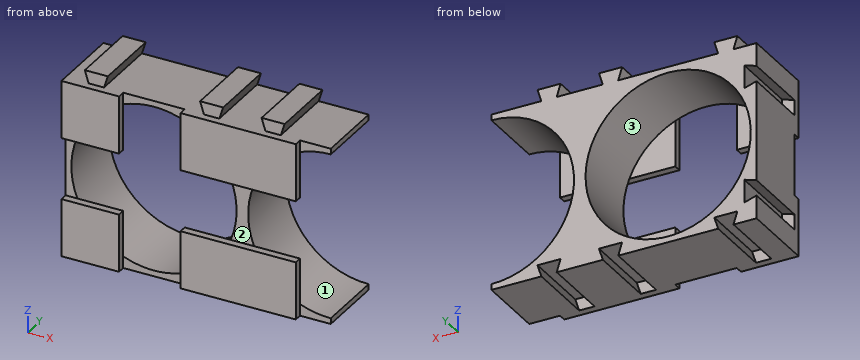
from build123d import *

# Parameters (mm, degrees)
SKETCH1_W           = 47.6
SKETCH1_H           = 24.6
BOSS_EXTRUDE1_DEPTH = 10
SKETCH2_R           = 10.75
CUT_EXTRUDE1_DEPTH  = 9
CUT_EXTRUDE2_DEPTH  = 9
SKETCH5_W           = 1.6
SKETCH5_H           = 24.6
CUT_EXTRUDE3_DEPTH  = 10
SKETCH6_W           = 46
SKETCH6_H           = 1.6
CUT_EXTRUDE4_DEPTH  = 10
BOSS_EXTRUDE2_DEPTH = 9
SKETCH10_W          = 46
SKETCH10_H          = 8.003908937
CUT_EXTRUDE5_DEPTH  = 1
SKETCH11_W          = 8
SKETCH11_H          = 23
CUT_EXTRUDE6_DEPTH  = 1
SKETCH12_W          = 13.355704333
SKETCH12_H          = 24.6
CUT_EXTRUDE8_DEPTH  = 10


with BuildPart() as part:
    # Sketch1 → Boss-Extrude1 (new body)
    with BuildSketch(Plane(origin=(0, 0, 0), x_dir=(1, 0, 0), z_dir=(0, 1, 0))):
        with Locations((23.8, 12.3)):
            Rectangle(SKETCH1_W, SKETCH1_H)
    extrude(amount=BOSS_EXTRUDE1_DEPTH)

    # Sketch2 → Cut-Extrude1 (cut)
    with BuildSketch(Plane(origin=(0, 10, 0), x_dir=(1, 0, 0), z_dir=(0, 1, 0))):
        with Locations(Location((11.5, 13.1, 0), (0, 0, 270))):
            Circle(SKETCH2_R)
        with Locations(Location((34.5, 13.1, 0), (0, 0, 270))):
            Circle(SKETCH2_R)
    extrude(amount=-CUT_EXTRUDE1_DEPTH, mode=Mode.SUBTRACT)

    # Sketch3 → Cut-Extrude2 (cut)
    with BuildSketch(Plane(origin=(0, 10, 0), x_dir=(1, 0, 0), z_dir=(0, 1, 0))):
        Polygon((3, 24.6), (2.5, 23), (5.5, 23), (5, 24.6), align=None)
        Polygon((18, 24.6), (17.5, 23), (20.5, 23), (20, 24.6), align=None)
        Polygon((26, 24.6), (25.5, 23), (28.5, 23), (28, 24.6), align=None)
        Polygon((41, 24.6), (40.5, 23), (43.5, 23), (43, 24.6), align=None)
        Polygon((0, 21.6), (1.6, 22.1), (1.6, 19.1), (0, 19.6), align=None)
        Polygon((0, 6.6), (1.6, 7.1), (1.6, 4.1), (0, 4.6), align=None)
    extrude(amount=-CUT_EXTRUDE2_DEPTH, mode=Mode.SUBTRACT)

    # Sketch5 → Cut-Extrude3 (cut)
    with BuildSketch(Plane(origin=(0, 10, 0), x_dir=(1, 0, 0), z_dir=(0, 1, 0))):
        with Locations((46.8, 12.3)):
            Rectangle(SKETCH5_W, SKETCH5_H)
    extrude(amount=-CUT_EXTRUDE3_DEPTH, mode=Mode.SUBTRACT)

    # Sketch6 → Cut-Extrude4 (cut)
    with BuildSketch(Plane(origin=(0, 10, 0), x_dir=(1, 0, 0), z_dir=(0, 1, 0))):
        with Locations((23, 0.8)):
            Rectangle(SKETCH6_W, SKETCH6_H)
    extrude(amount=-CUT_EXTRUDE4_DEPTH, mode=Mode.SUBTRACT)

    # Sketch7 → Boss-Extrude2 (add)
    with BuildSketch(Plane(origin=(0, 10, 0), x_dir=(1, 0, 0), z_dir=(0, 1, 0))):
        Polygon((46, 21.6), (47.6, 22.1), (47.6, 19.1), (46, 19.6), align=None)
        Polygon((46, 6.6), (47.6, 7.1), (47.6, 4.1), (46, 4.6), align=None)
        Polygon((3, 1.6), (2.5, 0), (5.5, 0), (5, 1.6), align=None)
        Polygon((18, 1.6), (17.5, 0), (20.5, 0), (20, 1.6), align=None)
        Polygon((26, 1.6), (25.5, 0), (28.5, 0), (28, 1.6), align=None)
        Polygon((41, 1.6), (40.5, 0), (43.5, 0), (43, 1.6), align=None)
    extrude(amount=-BOSS_EXTRUDE2_DEPTH)

    # Sketch10 → Cut-Extrude5 (cut)
    with BuildSketch(Plane.XZ):
        with Locations((23, -13.101954469)):
            Rectangle(SKETCH10_W, SKETCH10_H)
    extrude(amount=-CUT_EXTRUDE5_DEPTH, mode=Mode.SUBTRACT)

    # Sketch11 → Cut-Extrude6 (cut)
    with BuildSketch(Plane.XZ):
        with Locations((11.5, -13.1)):
            Rectangle(SKETCH11_W, SKETCH11_H)
        with Locations((34.5, -13.1)):
            Rectangle(SKETCH11_W, SKETCH11_H)
    extrude(amount=-CUT_EXTRUDE6_DEPTH, mode=Mode.SUBTRACT)

    # Sketch12 → Cut-Extrude8 (cut)
    with BuildSketch(Plane(origin=(0, 10, 0), x_dir=(1, 0, 0), z_dir=(0, 1, 0))):
        with Locations((41.177852167, 12.3)):
            Rectangle(SKETCH12_W, SKETCH12_H)
    extrude(amount=-CUT_EXTRUDE8_DEPTH, mode=Mode.SUBTRACT)


solid = part.part
Design review of the part built by this model. Coordinates are the model's own, in mm. Face numbers are marked on the shaded views. A direction names the side the tool comes from. Round coordinates to 2 decimals unless told otherwise and drop trailing zeros. Write each loop counter-clockwise with the first axis right and the second up, starting at its lowest first coordinate (ties: lowest second). Pieces come first, ordered by that corner, then holes.
Item 1: For the marked faces 1, 2 and 3, list the 3-axis set-ups (+Z, -Z, +X, -X, +Y, -Y) from which the entire face can be reached by the end or side of a thin tool; tool diameter is ignored.
Item 2: Consider section C-C on z = -1.25. Give the boundary of the cut face in (x, y), and give its area (3 significant figures).
Item 3: Wall thickness on L1, parallel to X at y = 5, z = -13.1; L2, parallel to X at y = 6, z = -17; L3, parallel to Z at x = 30.5, y = 6: over which ranges is each line inside the solid? List them lowest first.
Item 4: Consider section D-D on x = 6. Give the boundary of the cut face in (y, z), and give its area (3 significant figures).
Item 5: Consider section B-B on z = -13.1. Give the boundary of the cut face in (x, y), and give its area (4 significant figures).
Item 6: Consider section A-A on x = 11.5. Give the boundary of the cut face in (y, z).
Item 7: For pin 1 Ø1.5 at (x, z) = (22.5, -12) entering from -Y; pin 2 Ø0.5 at (x, z) = (0.5, -20.5) entering from +Y; pin 3 Ø0.5 at (y, z) = (0.5, -22) entering from +X; pin 4 Ø2 at (x, z) = (12.5, -4) entering from +Y, all flat-tipped, find the tip position at first contact; note any pin that passes through.
Check values:
1. face 1: +X, +Y
1. face 2: +X, -X, -Y
1. face 3: +Y
2. outline: (2.89, 1) - (5.11, 1) - (5.11, 10) - (2.89, 10) - close; (17.89, 1) - (20.11, 1) - (20.11, 10) - (17.89, 10) - close; (25.89, 1) - (28.11, 1) - (28.11, 10) - (25.89, 10) - close
2. area: 59.9 mm2
3. L1: x = 0 to 0.75, 22.25 to 23.75
3. L2: x = 0 to 1.48, 21.52 to 24.48
3. L3: z = -24.6 to -23.08, -3.12 to -1.6
4. outline: (0, -24.6) - (10, -24.6) - (10, -22.34) - (1, -22.34) - (1, -17.1) - (0, -17.1) - close; (0, -9.1) - (1, -9.1) - (1, -3.86) - (10, -3.86) - (10, -1.6) - (0, -1.6) - close
4. area: 55.7 mm2
5. outline: (0, 1) - (0.75, 1) - (0.75, 10) - (0, 10) - close; (22.25, 1) - (23.75, 1) - (23.75, 10) - (22.25, 10) - close
5. area: 20.25 mm2
6. outline: (1, -24.6) - (10, -24.6) - (10, -23.85) - (1, -23.85) - close; (1, -2.35) - (10, -2.35) - (10, -1.6) - (1, -1.6) - close
7. pin 1: stops at y = 1
7. pin 2: stops at y = 1
7. pin 3: stops at x = 30.5
7. pin 4: passes through
